Verification items for the finished model (mm, model axes). Face numbers are marked on the shaded views. A direction names the side the tool comes from. Round coordinates to 2 decimals unless told otherwise and drop trailing zeros. Loops run counter-clockwise (first coordinate to the right, second up) from the corner with the lowest first, then second, coordinate; pieces in that order, holes last. Notation, with made-up numbers: M 31,22.5 L 65,22.5 A28 cw 65,55.5 Z; hole C 9,22.25 d2. An arc over 180 degrees is marked long. Write item = value, one per line. Start each with the question number.
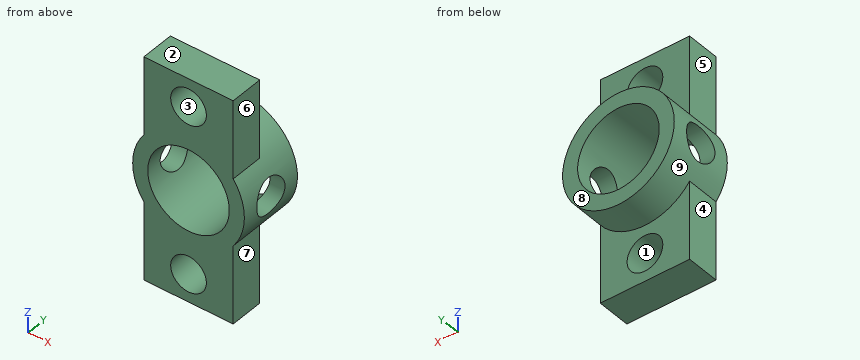
Autodesk Inventor part; units mm, degrees
ref_plane "Work Plane1" through (5, 0, 0) normal (1, 0, 0) x (0, 0, -1)
ref_plane "YZ Plane" through (0, 0, 0) normal (1, 0, 0) x (0, 1, 0)
ref_plane "XZ Plane" through (0, 0, 0) normal (0, 1, 0) x (-1, 0, 0)
sketch "Sketch1" plane through (0, 0, 0) normal (0, 1, 0) x (-1, 0, 0)
  circle A0 centre (0, 0) radius 3.65
  circle A1 centre (0, 0) radius 5
  line L0 (4, 10) -> (-4, 10)
  line L1 (-4, 10) -> (-4, -10)
  line L2 (-4, -10) -> (4, -10)
  line L3 (4, -10) -> (4, 10)
  line L4 (4, 10) -> (-4, -10) construction
  line L5 (-4, 10) -> (4, -10) construction
  circle A2 centre (0, 7.5) radius 1.6
  circle A3 centre (0, -7.5) radius 1.6
  point P0 (4, -3)
  point P1 (-4, -3)
  point P2 (4, 3)
  point P3 (-4, 3)
  dimension "d0" = 7.3
  dimension "d1" = 10
  dimension "d2" = 20
  dimension "d3" = 3.2
  dimension "d4" = 2.5
  dimension "d5" = 3.2
  dimension "d6" = 2.5
extrude "Extrusion1" add sketch "Sketch1" along normal blind 3 contours A1 L3 | A1 L1 L0 L3 | L3 L2 L1 A1 | L1 A1
extrude "Extrusion2" add sketch "Sketch1" along normal blind 6 contours A1 L3 | L3 A1 L1 | L1 A1
ref_plane "Work Plane1" through (5, 0, 0) normal (1, 0, 0) x (0, 0, -1)
sketch "Sketch2" plane through (5, 0, 0) normal (1, 0, 0) x (0, 0, -1)
  circle A0 centre (0, 3) radius 1.6
  point P0 (0, 0)
  dimension "d11" = 3.2
extrude "Extrusion3" cut sketch "Sketch2" against normal blind 10
properties part number "Fix Bracket Lifter"
1. Section check A-A, the plane z = -7.5. Enter the section's corners in (x, y), and give its area (3 significant figures).
2. Mould release check, pull along Z, two halves, no side actions. Record for the marked faces 1, 2, 3 and 4: pulls with the +Z half, pulls with the -Z half, needs draft (parallel to the pull), parting line crosses it, or undercut.
3. Gauge pin test, flat ends, axial feed: P1, Ø3.5, axis at y = 2, z = 6.5, coming from the -X side; P2, Ø2.5, axis at y = 3, z = 0, coming from the -X side; P3, Ø1.5, axis at y = 1.5, z = 7, coming from the +X side. Record the tip position at first contact, or that the pin passes through.
4. Section check C-C, the plane x = -0.5. Enter the section's corners in (y, z).
5. Tool access check on the marked faces 5, 6, 7, 8 and 9. Record the directions out of +Z, -Z, +X, -X, +Y, -Y that give a thin tool (end or side, any length) a straight path to the whole face; none if there is none.
6. Thickness scan on line 1 (Z direction, x = 0, y = 1.35); line 2 (X direction, y = 4.75, z = 0); line 3 (Y direction, x = -3.8, z = 0). Record the ranges inside material, lowest first.
7. Section check B-B, the plane y = 2.75. Enter the section's corners in (x, z), and give its area (3 significant figures).
Computed values:
q1.outline = M -4,0 L -1.6,0 L -1.6,3 L -4,3 Z; M 1.6,0 L 4,0 L 4,3 L 1.6,3 Z
q1.area = 14.4 mm2
q2.face_1 = undercut
q2.face_2 = pulls with the +Z half
q2.face_3 = undercut
q2.face_4 = needs draft
q3.P1 = -4
q3.P2 = through
q3.P3 = 4
q4.outline = M 0,-10 L 3,-10 L 3,-9.02 L 0,-9.02 Z; M 0,-5.98 L 3,-5.98 L 3,-4.97 L 6,-4.97 L 6,-3.62 L 0,-3.62 Z; M 0,3.62 L 6,3.62 L 6,4.97 L 3,4.97 L 3,5.98 L 0,5.98 Z; M 0,9.02 L 3,9.02 L 3,10 L 0,10 Z
q5.face_5 = +Z, -X, +Y, -Y
q5.face_6 = +Z, +X, +Y, -Y
q5.face_7 = -Z, +X, +Y, -Y
q5.face_8 = +Z, -Z, +X, -X, +Y
q5.face_9 = +Y
q6.line_1 = -10 to -9.1, -5.9 to -3.65, 3.65 to 5.9, 9.1 to 10
q6.line_2 = -5 to -3.65, 3.65 to 5
q6.line_3 = 0 to 1.4, 4.6 to 6
q7.outline = M -4.74,-1.58 A5 ccw -4,-3 L -4,-10 L 4,-10 L 4,-3 A5 ccw 4.74,-1.58 L 3.29,-1.58 A3.65 cw -3.29,-1.58 Z; M -4.74,1.58 L -3.29,1.58 A3.65 cw 3.29,1.58 L 4.74,1.58 A5 ccw 4,3 L 4,10 L -4,10 L -4,3 A5 ccw Z; hole C 0,-7.5 d3.2; hole C 0,7.5 d3.2
q7.area = 101 mm2
